Verification items for the finished model (mm, model axes). A direction names the side the tool comes from. Round coordinates to 2 decimals unless told otherwise and drop trailing zeros. Order: outer loops, then holes, each group sorted by start corner. A loop starts at its lowest first (then second) coordinate and runs counter-clockwise, first axis right, second up. Notation, with made-up numbers: (6.25, 49.5) -> (55.25, 49.5) arc R24 cw to (55.25, 64.5) -> close; hole circle Ø1 at (-7.75, 66). An arc over 180 degrees is marked (long way). Return JSON: item names as keys, results as strings. Group by question number.
Item 1: Sectioned sample at A-A on x = 0. Record the cut outline in (y, z).
Item 2: Access from +Z, -Z, +X, -X, +Y, -Y to the whole of each face (thin tool, end or side, straight path). Record for faces 1 (the flat face through (0, -3, -5)), 2 (the flat face through (0, -13, -2)), 3 (the cylindrical face through (-2.9, -9.09, -1.11)).
Item 3: Depth check by flat-ended pin: pin 1 Ø10 at (x, z) = (-2, 4) entering from +Y; pin 2 Ø2.5 at (x, z) = (0, -8) entering from -Y; pin 3 Ø2 at (y, z) = (-9.67, 0) entering from -X; pin 4 Ø5 at (x, y) = (-4, -9.5) entering from -Z. Enter the tip coordinate at first touch or a pass-through.
Item 4: Sectioned sample at B-B on z = 0. Record the cut outline in (x, y), plus the area to 3 significant figures.
Item 5: Sectioned sample at D-D on x = -3.5. Record the cut outline in (y, z), plus the area to 3 significant figures.
Item 6: Sectioned sample at C-C on z = -9. Record the cut outline in (x, y), plus the area to 3 significant figures.
Item 7: Draft check along X on faces 4 (the flat face through (0, 0, -3)), 5 (the cylindrical face through (4.34, -7.93, -1.8)), 6 (the cylindrical face through (1.57, -6.41, -0.65)). Enter one of: pulls with the +X half, pulls with the -X half, needs draft (parallel to the pull), parting line crosses it, or undercut.
Item 8: Scan lines: probe 1 along Z at (x, y) = (0, -2); probe 2 along Z at (x, y) = (0, -8.5). Record each from-to range of solid material in increasing order. Write a range as from..to.
```python
from build123d import *

# Parameters (mm, degrees)
F2_R     = 12.5
F2_R_2   = 1.5
F2_R_3   = 1.7
F3_DEPTH = 3
F4_R     = 4.7
F4_R_2   = 1.7
F5_DEPTH = 10
F6_R     = 1.25
F7_DEPTH = 25


with BuildPart() as f3:
    # F2 (on Front) → F3 (new body)
    with BuildSketch(Plane.XZ):
        Circle(F2_R)
        with Locations((0, -8)):
            Circle(F2_R_2, mode=Mode.SUBTRACT)
        Circle(F2_R_3, mode=Mode.SUBTRACT)
        with Locations((0, 8)):
            Circle(F2_R_2, mode=Mode.SUBTRACT)
    extrude(amount=F3_DEPTH)

    # F4 (on face) → F5 (join)
    with BuildSketch(Plane.XZ.offset(3)):
        Circle(F4_R)
        Circle(F4_R_2, mode=Mode.SUBTRACT)
    extrude(amount=F5_DEPTH)

    # F6 (on Right) → F7 (cut)
    with BuildSketch(Plane.YZ):
        with Locations((-9.6666666667, 0)):
            Circle(F6_R)
    extrude(amount=-F7_DEPTH, mode=Mode.SUBTRACT)


solid = f3.part
```
Recorded:
{
 "1": {"outline": "(-13, -4.7) -> (-3, -4.7) -> (-3, -6.5) -> (0, -6.5) -> (0, -1.7) -> (-13, -1.7) -> close; (-13, 1.7) -> (0, 1.7) -> (0, 6.5) -> (-3, 6.5) -> (-3, 4.7) -> (-13, 4.7) -> close; (-3, -12.5) -> (0, -12.5) -> (0, -9.5) -> (-3, -9.5) -> close; (-3, 9.5) -> (0, 9.5) -> (0, 12.5) -> (-3, 12.5) -> close"},
 "2": {"face 1": "-Y", "face 2": "+Z, -Z, +X, -X, -Y", "face 3": "-X"},
 "3": {"pin 1": "y = 0", "pin 2": "through", "pin 3": "x = 1.37", "pin 4": "z = -4.45"},
 "4": {"outline": "(-12.5, -3) -> (-4.7, -3) -> (-4.7, -8.42) -> (-1.7, -8.42) -> (-1.7, 0) -> (-12.5, 0) -> close; (-4.7, -13) -> (-1.7, -13) -> (-1.7, -10.92) -> (-4.7, -10.92) -> close; (1.7, -13) -> (4.7, -13) -> (4.7, -3) -> (12.5, -3) -> (12.5, 0) -> (1.7, 0) -> close", "area": "117 mm²"},
 "5": {"outline": "(-13, -3.14) -> (-3, -3.14) -> (-3, -12) -> (0, -12) -> (0, 12) -> (-3, 12) -> (-3, 3.14) -> (-13, 3.14) -> close; hole circle Ø2.5 at (-9.67, 0)", "area": "130 mm²"},
 "6": {"outline": "(-8.67, -3) -> (-1.12, -3) -> (-1.12, 0) -> (-8.67, 0) -> close; (1.12, -3) -> (8.67, -3) -> (8.67, 0) -> (1.12, 0) -> close", "area": "45.3 mm²"},
 "7": {"face 4": "needs draft", "face 5": "parting line crosses it", "face 6": "undercut"},
 "8": {"probe 1": "-12.5..-9.5, -6.5..-1.7, 1.7..6.5, 9.5..12.5", "probe 2": "-4.7..-1.7, 1.7..4.7"}
}
